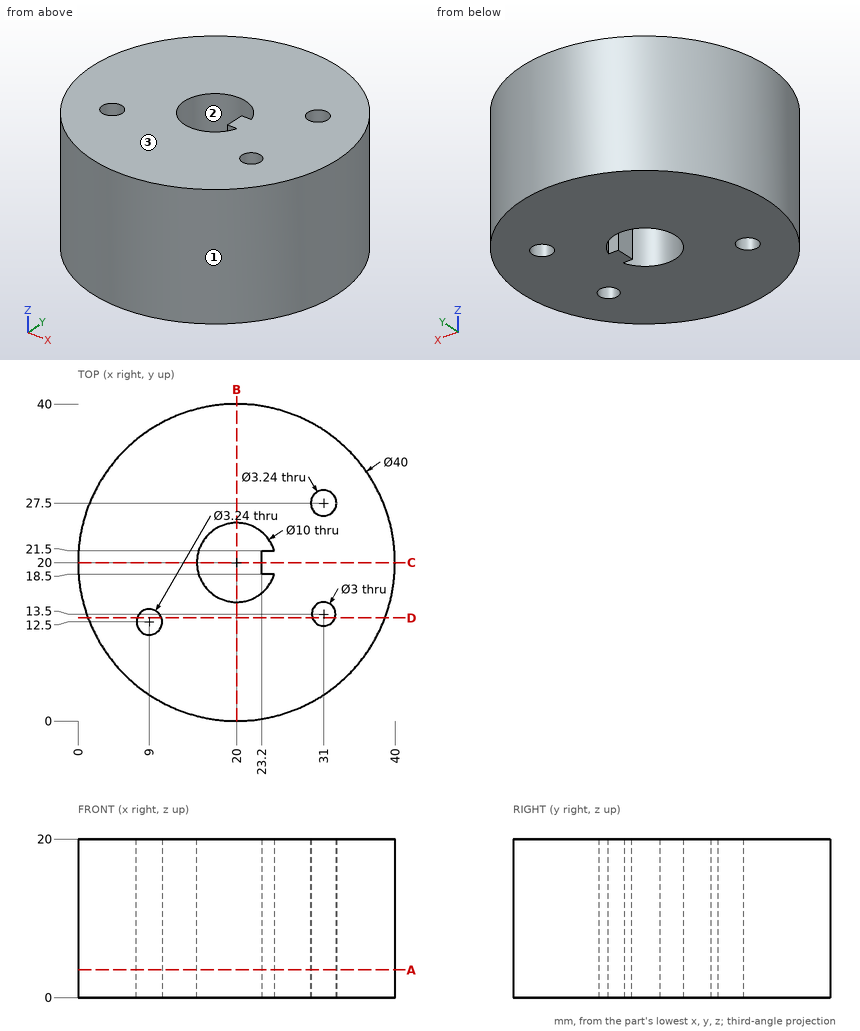
Geometry check sheet. Reference: drawing and pictorial views, mm from the part's lowest x, y, z. Give positions to 0.01 mm unless a question says otherwise; leave off trailing zeros. Write each loop counter-clockwise with the first axis right and the second up, starting at its lowest first coordinate (ties: lowest second). Pieces come first, ordered by that corner, then holes. Notation, with made-up numbers: (11, 58.5) - (30, 58.5) arc R19 cw to (30, 63.5) - close; hole circle Ø2 at (34.5, 84.5). An arc over 180 degrees is marked (long way). Put each result on its own line as item: value.
Q1. Scan lines: probe 1 along Y at (x, z) = (20, 11); probe 2 along Y at (x, z) = (31, 10.5); probe 3 along Y at (x, z) = (24.5, 5). Record each from-to range of solid material in increasing order. Write a range as from..to.
Result:
probe 1: 0..15, 25..40
probe 2: 3.3..12, 15..25.88, 29.12..36.7
probe 3: 0.51..17.82, 18.5..21.5, 22.18..39.49
Q2. Section check C-C on y = 20. Record the cut outline in (x, z).
Result:
outline: (0, 0) - (15, 0) - (15, 20) - (0, 20) - close; (23.2, 0) - (40, 0) - (40, 20) - (23.2, 20) - close
Q3. Section check D-D on y = 13. Record the cut outline in (x, z) (3 decimals).
Result:
outline: (1.265, 0) - (7.459, 0) - (7.459, 20) - (1.265, 20) - close; (10.541, 0) - (29.586, 0) - (29.586, 20) - (10.541, 20) - close; (32.414, 0) - (38.735, 0) - (38.735, 20) - (32.414, 20) - close
Q4. Section check B-B on x = 20. Record the cut outline in (y, z), and give its area (3 significant figures).
Result:
outline: (0, 0) - (15, 0) - (15, 20) - (0, 20) - close; (25, 0) - (40, 0) - (40, 20) - (25, 20) - close
area: 600 mm2
Q5. Depth check by flat-ended pin: P1, Ø0.5, axis at x = 24, z = 10.5, coming from the +Y side; P2, Ø0.5, axis at x = 24.5, z = 12.5, coming from the -Y side; P3, Ø1.9, axis at x = 31, y = 27.5, coming from the +Z side; P4, Ø10, axis at y = 6, z = 5, coming from the -X side. Enter the tip coordinate at first touch or a pass-through.
Result:
P1: y = 39.65
P2: y = 0.46
P3: through
P4: x = 2.14
Q6. Mould release check, pull along Y, two halves, no side actions. Record for the marked faces 1, 2 and 3: released by +Y, released by -Y, zero draft, split by the parting line, or undercut.
Result:
face 1: split by the parting line
face 2: undercut
face 3: zero draft
Q7. Section check A-A on z = 3.5. Record the cut outline in (x, y).
Result:
outline: circle Ø40 at (20, 20); hole circle Ø3.24 at (9, 12.5); hole (23.2, 18.5) - (23.2, 21.5) - (24.77, 21.5) arc R5 ccw (long way) to (24.77, 18.5) - close; hole circle Ø3.24 at (31, 27.5); hole circle Ø3 at (31, 13.5)
